Design review of the part built by this model. Coordinates are the model's own, in mm. A direction names the side the tool comes from. Give positions to 0.01 mm unless a question says otherwise; leave off trailing zeros. Write each loop counter-clockwise with the first axis right and the second up, starting at its lowest first coordinate (ties: lowest second). Pieces come first, ordered by that corner, then holes. Notation, with made-up numbers: M 39.25,57.25 L 66.25,57.25 A9 cw 66.25,62.25 Z; hole C -9,-10.75 d11. An arc over 180 degrees is marked long. Answer in a Markdown table with one row per item.
```python
from build123d import *

# Parameters (mm, degrees)
SKETCH_2_W          = 70
SKETCH_2_H          = 80
SKETCH_2_R          = 23.5
SKETCH_2_R_2        = 1.6
EXTRUDE_4_DEPTH     = 12
SKETCH_6_W          = 80
SKETCH_6_H          = 40
EXTRUDE_6_DEPTH     = 5
FILLET_3_R          = 5
FILLET_4_R          = 5
FILLET_5_R          = 5
FILLET_6_R          = 5
SKETCH_7_R          = 1.5
CUT_EXTRUDE_4_DEPTH = 5
CUT_EXTRUDE_START   = -12
CUT_EXTRUDE_6_DEPTH = 12
FILLET_7_R          = 10
FILLET_8_R          = 10


with BuildPart() as part:
    # 草图2 → 凸台-拉伸4 (new body)
    with BuildSketch(Plane(origin=(0, 0, 0), x_dir=(1, 0, 0), z_dir=(0, 1, 0))):
        Rectangle(SKETCH_2_W, SKETCH_2_H)
        with Locations(Location((0, 0, 0), (0, 0, 270))):
            Circle(SKETCH_2_R, mode=Mode.SUBTRACT)
        with Locations(Location((-27.5, 27.5, 0), (0, 0, 270))):
            Circle(SKETCH_2_R_2, mode=Mode.SUBTRACT)
        with Locations(Location((27.5, 27.5, 0), (0, 0, 270))):
            Circle(SKETCH_2_R_2, mode=Mode.SUBTRACT)
        with Locations(Location((27.5, -27.5, 0), (0, 0, 270))):
            Circle(SKETCH_2_R_2, mode=Mode.SUBTRACT)
        with Locations(Location((-27.5, -27.5, 0), (0, 0, 270))):
            Circle(SKETCH_2_R_2, mode=Mode.SUBTRACT)
    extrude(amount=EXTRUDE_4_DEPTH)

    # 草图6 → 凸台-拉伸6 (add)
    with BuildSketch(Plane(origin=(0, 0, -40), x_dir=(-1, 0, 0), z_dir=(0, 0, -1))):
        with Locations((0, 6)):
            Rectangle(SKETCH_6_W, SKETCH_6_H)
    extrude(amount=EXTRUDE_6_DEPTH)

    # 圆角3
    fillet_3_edges = [part.edges().sort_by_distance(p)[0] for p in [
        (0, 12, -40),
    ]]
    fillet(fillet_3_edges, radius=FILLET_3_R)

    # 圆角4
    fillet_4_edges = [part.edges().sort_by_distance(p)[0] for p in [
        (0, 0, -40),
    ]]
    fillet(fillet_4_edges, radius=FILLET_4_R)

    # 圆角5
    fillet_5_edges = [part.edges().sort_by_distance(p)[0] for p in [
        (35, 6, -40),
    ]]
    fillet(fillet_5_edges, radius=FILLET_5_R - 0.0001)  # a hair under: the kernel refuses the full size

    # 圆角6
    fillet_6_edges = [part.edges().sort_by_distance(p)[0] for p in [
        (-35, 6, -40),
    ]]
    fillet(fillet_6_edges, radius=FILLET_6_R - 0.0001)  # a hair under: the kernel refuses the full size

    # 草图7 → 切除-拉伸4 (cut)
    with BuildSketch(Plane.XY.offset(-40)):
        with Locations((-35, -9)):
            Circle(SKETCH_7_R)
        with Locations(Location((-35, 21, 0), (0, 0, 180))):
            Circle(SKETCH_7_R)
        with Locations(Location((35, -9, 0), (0, 0, 180))):
            Circle(SKETCH_7_R)
        with Locations((35, 21)):
            Circle(SKETCH_7_R)
    extrude(amount=-CUT_EXTRUDE_4_DEPTH, mode=Mode.SUBTRACT)

    # 草图8 → 切除-拉伸6 (cut)
    with BuildSketch(Plane(origin=(0, 12, 0), x_dir=(1, 0, 0), z_dir=(0, 1, 0)).offset(CUT_EXTRUDE_START)):
        with BuildLine():
            Line((0, -38.461215902), (0, -23.5))
            ThreePointArc((0, -23.5), (-10.095935407, -21.220793771), (-18.233511761, -14.825284107))
            Line((-18.233511761, -14.825284107), (0, -38.461215902))
        make_face()
        with BuildLine():
            ThreePointArc((18.233511761, -14.825284107), (10.095935407, -21.220793771), (0, -23.5))
            Line((0, -23.5), (0, -38.461215902))
            Line((0, -38.461215902), (18.233511761, -14.825284107))
        make_face()
    extrude(amount=CUT_EXTRUDE_6_DEPTH, mode=Mode.SUBTRACT)

    # 圆角7
    fillet_7_edges = [part.edges().sort_by_distance(p)[0] for p in [
        (-35, 6, 40),
    ]]
    fillet(fillet_7_edges, radius=FILLET_7_R)

    # 圆角8
    fillet_8_edges = [part.edges().sort_by_distance(p)[0] for p in [
        (35, 6, 40),
    ]]
    fillet(fillet_8_edges, radius=FILLET_8_R)


solid = part.part
```
1) Add section C-C (x = -13). Write out the cut boundary in (y, z), and give its area (3 significant figures).
Geometry says:
| item | result |
|---|---|
| outline | M -14,-45 L 26,-45 L 26,-40 L 17,-40 A5 cw 12,-35 L 12,-19.58 L 0,-19.58 L 0,-35 A5 cw -5,-40 L -14,-40 Z; M 0,21.61 L 12,21.61 L 12,40 L 0,40 Z |
| area | 676 mm^2 |
2) The part is to be moulded in two halves that separate along Z. For faces 1 (the face through (-25.914, 5.916, -27.708)), 2 (the face through (-24, 0, 2)), 3 (the face through (1, -2, -39)), say which applies: released by +Z, released by -Z, zero draft, split by the parting line, or undercut.
Geometry says:
| item | result |
|---|---|
| face 1 | undercut |
| face 2 | zero draft |
| face 3 | released by +Z |
3) Add section B-B (z = 24). Write out the cut boundary in (x, y).
Geometry says:
| item | result |
|---|---|
| outline | M -35,0 L -11.16,0 L -11.16,12 L -35,12 Z; M 11.16,0 L 35,0 L 35,12 L 11.16,12 Z |
4) To check wall thickness, follow probe 1 along X at (y, z) = (4.5, -27.5); probe 2 along Y at (x, z) = (35, -42.35); probe 3 along Z at (x, y) = (-27, 8). State the ranges of each line that lie inside material, in increasing order. Write a range as [from, to].
Geometry says:
| item | result |
|---|---|
| probe 1 | [-35, -29.1], [-25.9, 25.9], [29.1, 35] |
| probe 2 | [-14, -10.5], [-7.5, 19.5], [22.5, 26] |
| probe 3 | [-45, -29.02], [-25.98, 25.98], [29.02, 39.8] |
5) For faces 4 (the face through (1, -7, -40)), 5 (the face through (35, 6, -2)), 6 (the face through (-9.244, 5.916, 26.478)), 7 (the face through (-35, 6, -2)), 8 (the face through (-24, 12, 2)), list the 3-axis set-ups (+Z, -Z, +X, -X, +Y, -Y) from which the entire face can be reached by the end or side of a thin tool; tool diameter is ignored.
Geometry says:
| item | result |
|---|---|
| face 4 | +Z, +X, -X |
| face 5 | +Z, +X, +Y, -Y |
| face 6 | +Y, -Y |
| face 7 | +Z, -X, +Y, -Y |
| face 8 | +Z, +X, -X, +Y |
6) Add section D-D (z = -27.5). Write out the cut boundary in (x, y).
Geometry says:
| item | result |
|---|---|
| outline | M -35,0 L -29.1,0 L -29.1,12 L -35,12 Z; M -25.9,0 L 25.9,0 L 25.9,12 L -25.9,12 Z; M 29.1,0 L 35,0 L 35,12 L 29.1,12 Z |
7) Add section A-A (y = -9). Write out the cut boundary in (x, z).
Geometry says:
| item | result |
|---|---|
| outline | M -40,-45 L -36.5,-45 L -36.5,-40 L -40,-40 Z; M -33.5,-45 L 33.5,-45 L 33.5,-40 L -33.5,-40 Z; M 36.5,-45 L 40,-45 L 40,-40 L 36.5,-40 Z |
8) Insertion check: P1, Ø3, axis at y = 0.5, z = -23, coming from the -X side; P2, Ø3, axis at x = 23, z = -15, coming from the +Y side; P3, Ø5, axis at x = 27.5, z = 27.5, coming from the -Y side. Each pin has a flat end and moves straight along its axis. Give the tip position at first contact, or say it passes through.
Geometry says:
| item | result |
|---|---|
| P1 | x = -35 |
| P2 | y = 12 |
| P3 | y = 0 |
